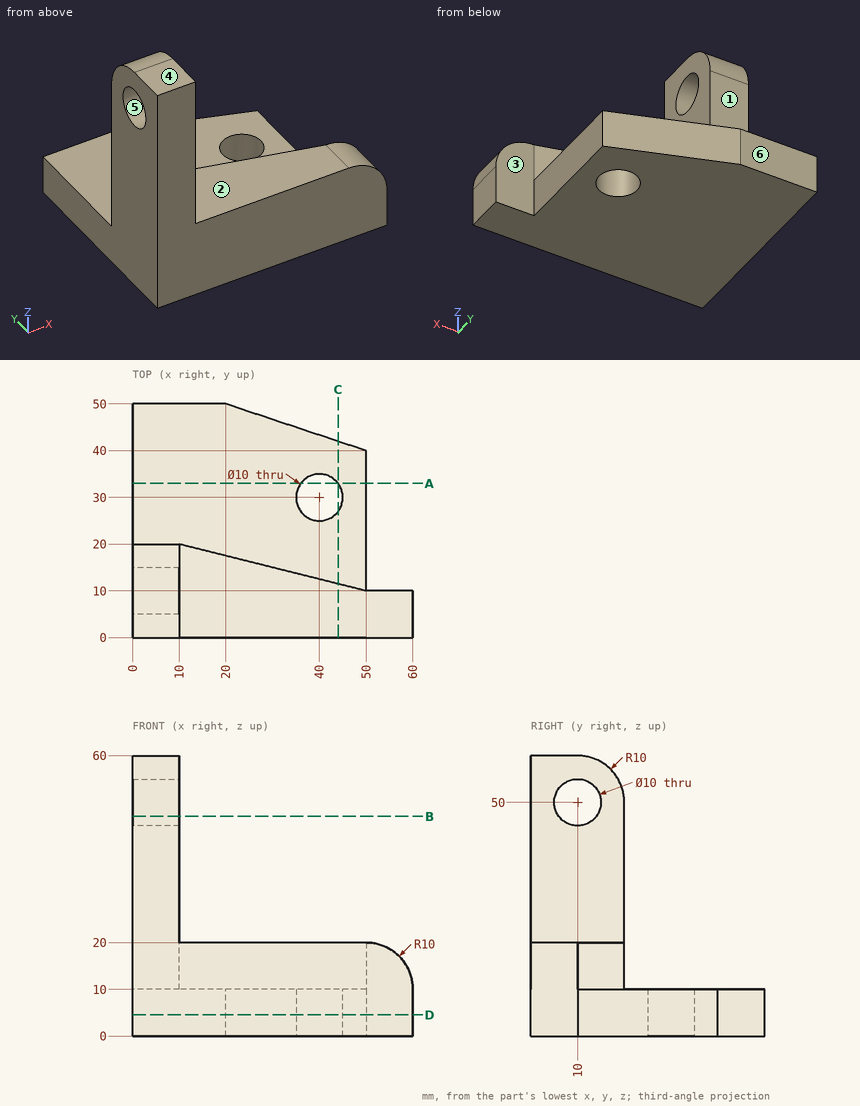
Part print with two shaded views. Sizes in mm from the minimum x, y, z corner. A direction names the side the tool comes from. Round coordinates to 2 decimals unless told otherwise and drop trailing zeros. Order: outer loops, then holes, each group sorted by start corner. A loop starts at its lowest first (then second) coordinate and runs counter-clockwise, first axis right, second up. Notation, with made-up numbers: M -2,41.25 L 17,41.25 A20 ccw 17,69.25 Z; hole C 27,2.25 d10. An arc over 180 degrees is marked long. Use CSV: the item, a comma, the result in double quotes. Start each with the question number.
(1) Cut at A-A on y = 33. List the corners of the cut face in (x, z), then the cut area to 3 significant figures.
(2) Cut at C-C on x = 44. List the corners of the cut face in (y, z), then the cut area to 3 significant figures.
(3) Tool access for the marked faces 1, 2 and 3: list every direction of +Z, -Z, +X, -X, +Y, -Y with a clear straight run to the whole face (end or side of a thin tool).
(4) Cut at B-B on z = 47. List the corners of the cut face in (x, y), then the cut area to 3 significant figures.
(5) Mould opens along Z. For the marked faces 4, 5 and 6 say: +Z half, -Z half, draft (parallel to the pull), parting line (faces both ways), or undercut.
(6) Cut at D-D on z = 4.5. List the corners of the cut face in (x, y), then the cut area to 3 significant figures.
(7) Flat gauge pins, fed straight in: P1, Ø16, axis at y = 10, z = 46.5, coming from the +X side; P2, Ø3, axis at y = 28, z = 3, coming from the +X side; P3, Ø20, axis at x = 35, y = 26, coming from the +Z side; P4, Ø10, axis at x = 24, z = 25.5, coming from the +Y side. Where does each tip first touch, or does it go through?
(8) Drill centre lines: probe 1 along Y at (x, z) = (5, 50); probe 2 along Z at (x, y) = (23, 43.5); probe 3 along Z at (x, y) = (15.5, 8.5). Where is each one in solid material? Low to high.
Findings:
1,outline,"M 0,0 L 36,0 L 36,10 L 0,10 Z; M 44,0 L 50,0 L 50,10 L 44,10 Z"
1,area,"420 mm^2"
2,outline,"M 0,0 L 27,0 L 27,10 L 11.5,10 L 11.5,20 L 0,20 Z; M 33,0 L 42,0 L 42,10 L 33,10 Z"
2,area,"475 mm^2"
3,face 1,"+Z, +X, -X, +Y"
3,face 2,"+Z, +X, +Y, -Y"
3,face 3,"+Z, -Z, +X, +Y"
4,outline,"M 0,0 L 10,0 L 10,6 L 0,6 Z; M 0,14 L 10,14 L 10,20 L 0,20 Z"
4,area,"120 mm^2"
5,face 4,"+Z half"
5,face 5,"undercut"
5,face 6,"draft"
6,outline,"M 0,0 L 60,0 L 60,10 L 50,10 L 50,40 L 20,50 L 0,50 Z; hole C 40,30 d10"
6,area,"2,370 mm^2"
7,P1,"stops at x = 10"
7,P2,"stops at x = 50"
7,P3,"stops at z = 10"
7,P4,"passes through"
8,probe 1,"y = 0 to 5, 15 to 20"
8,probe 2,"z = 0 to 10"
8,probe 3,"z = 0 to 20"
